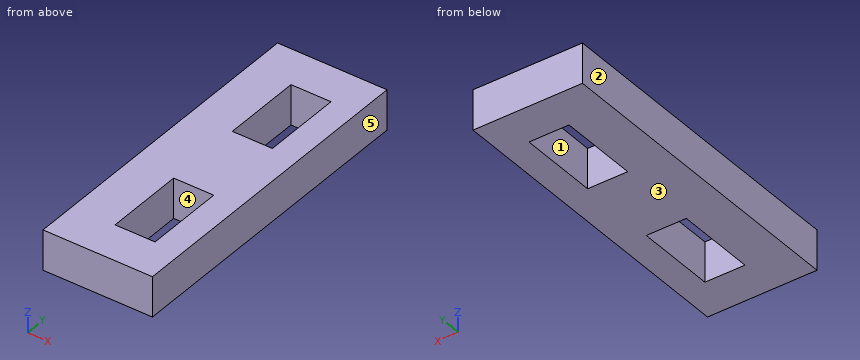
Autodesk Inventor part; units mm, degrees
ref_plane "YZ Plane" through (0, 0, 0) normal (1, 0, 0) x (0, 1, 0)
ref_plane "XZ Plane" through (0, 0, 0) normal (0, 1, 0) x (-1, 0, 0)
ref_plane "XY Plane" through (0, 0, 0) normal (0, 0, 1) x (1, 0, 0)
sketch "Sketch1" plane through (0, 0, 0) normal (0, 0, 1) x (1, 0, 0)
  line L0 (0, 0) -> (8.2022, 0)
  line L1 (8.2022, 0) -> (8.2022, 24)
  line L2 (8.2022, 24) -> (0, 24)
  line L3 (0, 24) -> (0, 0)
  line L4 (6.2022, 21) -> (3.2022, 21)
  line L5 (3.2022, 21) -> (3.2022, 15)
  line L6 (3.2022, 15) -> (6.2022, 15)
  line L7 (6.2022, 15) -> (6.2022, 21)
  line L8 (10.1659, 12) -> (-5.2678, 12)
  line L9 (6.2022, 3) -> (3.2022, 3)
  line L10 (3.2022, 3) -> (3.2022, 9)
  line L11 (3.2022, 9) -> (6.2022, 9)
  line L12 (6.2022, 9) -> (6.2022, 3)
  dimension "d0" = 24
  dimension "d1" = 3
  dimension "d2" = 6
  dimension "d3" = 3
  dimension "d4" = 2
extrude "Extrusion1" add sketch "Sketch1" along normal blind 3
equation "\"d0\" = CameraHeight"
equation "\"d1\" = Acrylic"
equation "\"d2\" = 0.25 * CameraHeight"
equation "\"d5\" = Acrylic"
equation "\"Acrylic\" = 3"
equation "\"CameraHeight\" = 24"
equation "\"CameraWidth\" = 25"
properties part number "SideClip"
Could you check a few things on this model? Use its own coordinates, in mm. Face numbers are marked on the shaded views. A direction names the side the tool comes from. Coordinates: 2 decimals unless noted, no trailing zeros. Order: outer loops, then holes, each group sorted by start corner. A loop starts at its lowest first (then second) coordinate and runs counter-clockwise, first axis right, second up. Notation, with made-up numbers: M -12,19.25 L -3,19.25 A23 cw -3,34.25 Z; hole C 20,86.25 d1. An arc over 180 degrees is marked long. Use a Markdown table: item, result. Add a question column.
Q1. I want a section at A-A on x = 5.75. List the corners of the cut face in (y, z) for me.
Q2. Which directions (+Z, -Z, +X, -X, +Y, -Y) give clear straight access to the entire face, cutting with the end or side of a thin tool? Please do the marked faces 1 and 2.
Q3. We'd pull the mould along X, two halves only. Please class the marked faces 3, 4 and 5: pulls with the +X half, pulls with the -X half, needs draft (parallel to the pull), parting line crosses it, or undercut.
Q4. I want a section at C-C on z = 1.05. List the corners of the cut face in (x, y) for me.
Q5. If I drill on L1, parallel to Y at x = 4.5, z = 0.7; L2, parallel to X at y = 19, z = 2.45, over which ranges is the centre line in solid material (lowest first)?
Q6. I want a section at B-B on y = 6.75. List the corners of the cut face in (x, z) for me, then the cut area to 3 significant figures.
Q7. I'm going to push a flat-ended pin straight in: pin 1 (3 mm diameter, centred on x = 6.5, y = 9, fed in from -Z). Where does the tip first touch, or does it pass through?
Checked values:
| question | item | result |
|---|---|---|
| 1 | outline | M 0,0 L 3,0 L 3,3 L 0,3 Z; M 9,0 L 15,0 L 15,3 L 9,3 Z; M 21,0 L 24,0 L 24,3 L 21,3 Z |
| 2 | face 1 | +Z, -Z |
| 2 | face 2 | +Z, -Z, -X, +Y, -Y |
| 3 | face 3 | needs draft |
| 3 | face 4 | undercut |
| 3 | face 5 | pulls with the +X half |
| 4 | outline | M 0,0 L 8.2,0 L 8.2,24 L 0,24 Z; hole M 3.2,3 L 6.2,3 L 6.2,9 L 3.2,9 Z; hole M 3.2,15 L 6.2,15 L 6.2,21 L 3.2,21 Z |
| 5 | L1 | 0 to 3, 9 to 15, 21 to 24 |
| 5 | L2 | 0 to 3.2, 6.2 to 8.2 |
| 6 | outline | M 0,0 L 3.2,0 L 3.2,3 L 0,3 Z; M 6.2,0 L 8.2,0 L 8.2,3 L 6.2,3 Z |
| 6 | area | 15.6 mm² |
| 7 | pin 1 | z = 0 |
